The model under review builds one solid part; all positions refer to its coordinate system, in mm. Coordinates: 2 decimals unless noted, no trailing zeros. Order: outer loops, then holes, each group sorted by start corner. A loop starts at its lowest first (then second) coordinate and runs counter-clockwise, first axis right, second up. Notation, with made-up numbers: (4.5, -36.75) - (38.5, -36.75) arc R26 ccw to (38.5, -21.75) - close; hole circle Ø10 at (3.25, 36.25). An arc over 180 degrees is marked (long way). Answer in a Markdown table with one row per item.
```python
from build123d import *


with BuildPart() as part:
    # Sketch3 → Revolve1 (revolve)
    with BuildSketch(Plane.XY, mode=Mode.PRIVATE) as revolve1_sk:
        with BuildLine():
            Line((-76.2, 17.78), (-76.2, 11.43))
            Line((-76.2, 11.43), (-15.663873033, 11.43))
            Line((-15.663873033, 11.43), (-15.663873033, 0))
            Line((-15.663873033, 0), (-5.821373033, 0))
            Line((-5.821373033, 0), (1.798626967, 0))
            Line((1.798626967, 0), (1.798626967, 7.9375))
            Line((1.798626967, 7.9375), (-5.821373033, 7.9375))
            Line((-5.821373033, 7.9375), (-15.198905048, 17.315032015))
            ThreePointArc((-15.198905048, 17.315032015), (-15.713927115, 17.659158758), (-16.321437064, 17.78))
            Line((-16.321437064, 17.78), (-76.2, 17.78))
        make_face()
    revolve(revolve1_sk.sketch.rotate(Axis((24.172114646, 0, 0), (-1, 0, 0)), 90), axis=Axis((24.172114646, 0, 0), (-1, 0, 0)))


solid = part.part
```
Item 1: Clearance check with flat-ended pins moving along their axes: pin 1 Ø4 at (x, y) = (-21.5, 10) entering from +Z; pin 2 Ø12 at (x, z) = (-67, -9) entering from +Y; pin 3 Ø8 at (x, y) = (-15, -11) entering from -Z. State where each tip first meets the part, or that it passes through.
Check values:
| item | result |
|---|---|
| pin 1 | z = 15.88 |
| pin 2 | y = 17.53 |
| pin 3 | z = -16.26 |
Item 2: To check wall thickness, follow line 1 (Y direction, x = -28, z = 0); line 2 (X direction, y = -2.5, z = 1); line 3 (Z direction, x = -29, y = -4.5). State the ranges of each line that lie inside material, in increasing order. Write a range as from..to.
Check values:
| item | result |
|---|---|
| line 1 | -17.78..-11.43, 11.43..17.78 |
| line 2 | -15.66..1.8 |
| line 3 | -17.2..-10.51, 10.51..17.2 |
Item 3: We need section C-C, the plane x = -42. Write out the cut boundary in (y, z), then the cut area to 3 significant figures.
Check values:
| item | result |
|---|---|
| outline | circle Ø35.56 at (0, 0); hole circle Ø22.86 at (0, 0) |
| area | 583 mm^2 |
Item 4: Mouldability with a two-part tool opening along Z and no side actions: class faces 1 (the face through (-2.06, 7.75, 1.72)), 2 (the face through (-15.664, 0, 0)), 3 (the face through (-45.508, 6.955, 9.07)), 4 (the face through (-76.2, 12, 0)) as +Z half, -Z half, draft (parallel to the pull), parting line (faces both ways), or undercut.
Check values:
| item | result |
|---|---|
| face 1 | parting line |
| face 2 | undercut |
| face 3 | undercut |
| face 4 | draft |
Item 5: We need section A-A, the plane z = 0. Write out the cut boundary in (x, y) (1 decimal), then the cut area to 3 significant figures.
Check values:
| item | result |
|---|---|
| outline | (-76.2, -17.8) - (-16.3, -17.8) arc R1.6 ccw to (-15.2, -17.3) - (-5.8, -7.9) - (1.8, -7.9) - (1.8, 7.9) - (-5.8, 7.9) - (-15.2, 17.3) arc R1.6 ccw to (-16.3, 17.8) - (-76.2, 17.8) - (-76.2, 11.4) - (-15.7, 11.4) - (-15.7, -11.4) - (-76.2, -11.4) - close |
| area | 1,140 mm^2 |
